The listing builds one solid part. Answer for the finished solid, in the listing's coordinates (mm). Face numbers are marked on the shaded views. A direction names the side the tool comes from. Coordinates: 2 decimals unless noted, no trailing zeros. Order: outer loops, then holes, each group sorted by start corner. A loop starts at its lowest first (then second) coordinate and runs counter-clockwise, first axis right, second up. Notation, with made-up numbers: M 43,6.5 L 90,6.5 A28 ccw 90,31.5 Z; hole C -33,38 d2. An arc over 180 degrees is marked long. One line per item, written item: value. Start each with the question number.
Q1. The part is cut by section B-B on z = -66. Give the vertices of the cut face in (x, y).
Q2. For the marked faces 1 and 2, determine the directions among +Z, -Z, +X, -X, +Y, -Y from which every point of the face is accessible in a straight line to the end or side of a thin tool.
Q3. The part is cut by section A-A on y = 0. Give the vertices of the cut face in (x, z) (1 decimal).
Q4. Straight lines are drawn through the part: line 1 along Z through (x, y) = (0.75, 8.75); line 2 along Y through (x, z) = (3, -17.5); line 3 along X through (y, z) = (2.5, -50.5). For each, find the intervals that lie inside material, in ascending order. Write a range as [from, to].
Q5. The part is cut by section C-C on y = -6.25. Give the vertices of the cut face in (x, z), then the cut area to 3 significant figures.
Q6. Each of these flat-tipped pins is pushed along its axis until it touches: pin 1 Ø6 at (x, z) = (-3.5, -3.5) entering from +Y; pin 2 Ø3 at (x, z) = (4, -17.5) entering from -Y; pin 3 Ø4.5 at (x, z) = (0, -1) entering from -Y (3 decimals). Where does it stop, or does it pass through?
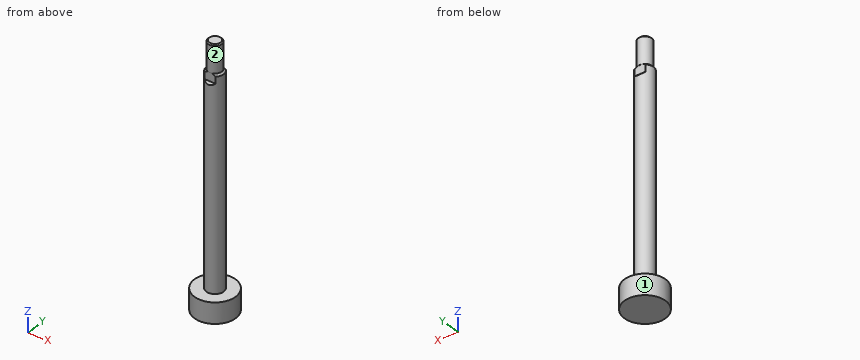
Autodesk Inventor part; units mm, degrees
ref_plane "conn_XY" through (0, 0, 0) normal (0, 0, -1) x (1, 0, 0)
ref_plane "conn_YZ" through (0, 0, 0) normal (1, 0, 0) x (0, -1, 0)
ref_plane "conn_ZX" through (0, 0, 0) normal (0, -1, 0) x (0, 0, -1)
sketch "Sketch_1" plane through (0, 0, 0) normal (1, 0, 0) x (0, 1, 0)
  line L0 (0, -106.5721) -> (0, 12.7)
  line L1 (0, 12.7) -> (2.634, 12.7)
  line L2 (2.634, 12.7) -> (3.175, 12.159)
  line L3 (3.175, 12.159) -> (3.175, 0)
  line L4 (3.175, 0) -> (4.0005, -0.8255)
  line L5 (4.0005, -0.8255) -> (4.0005, -97.0471)
  line L6 (4.0005, -97.0471) -> (9.5123, -97.0471)
  line L7 (9.5123, -97.0471) -> (9.5123, -106.5721)
  line L8 (9.5123, -106.5721) -> (0, -106.5721)
  line L9 (0, -106.5721) -> (0, 12.7)
revolve "Revolution1" add sketch "Sketch_1" angle 360 about axis through (0, 0, -106.5721) along (0, 0, -1)
thread "Thread1"
sketch "Sketch_2" plane through (0, 0, 0) normal (1, 0, 0) x (0, 1, 0)
  line L0 (6.096, 0) -> (3.048, 0)
  line L1 (3.048, 0) -> (3.048, -3.9878)
  line L2 (3.048, -3.9878) -> (6.096, -7.0358)
  line L3 (6.096, -7.0358) -> (6.096, 0)
extrude "Extrusion1" cut sketch "Sketch_2" along normal mid plane 16.002
sketch "Sketch_3" plane through (0, 0, 0) normal (1, 0, 0) x (0, 1, 0)
  line L0 (-6.096, 0) -> (-6.096, -7.0358)
  line L1 (-6.096, -7.0358) -> (-3.048, -3.9878)
  line L2 (-3.048, -3.9878) -> (-3.048, 0)
  line L3 (-3.048, 0) -> (-6.096, 0)
extrude "Extrusion2" cut sketch "Sketch_3" along normal mid plane 16.002
ref_plane "conn_XY" through (0, 0, 0) normal (0, 0, -1) x (1, 0, 0)
ref_plane "conn_YZ" through (0, 0, 0) normal (1, 0, 0) x (0, -1, 0)
ref_plane "conn_ZX" through (0, 0, 0) normal (0, -1, 0) x (0, 0, -1)
properties part number "PR_OCG1-3/4x2" material "Stainless Steel"
Output:
1. outline: C 0,0 d8
2. face 1: +Z, -Z
2. face 2: +Z
3. outline: M -9.5,-106.6 L 9.5,-106.6 L 9.5,-97 L 4,-97 L 4,-0.8 L 3.2,0 L 3.2,12.2 L 2.6,12.7 L -2.6,12.7 L -3.2,12.2 L -3.2,0 L -4,-0.8 L -4,-97 L -9.5,-97 Z
4. line 1: z = [-106.57, -97.05]
4. line 2: y = [-2.65, 2.65]
4. line 3: x = [-3.12, 3.12]
5. outline: M -7.17,-106.57 L 7.17,-106.57 L 7.17,-97.05 L -7.17,-97.05 Z
5. area: 137 mm^2
6. pin 1: stops at y = 3.91
6. pin 2: stops at y = -3.12
6. pin 3: stops at y = -3.175
